from build123d import *

# Parameters (mm, degrees)
EXTRUDE_1_DEPTH     = 300
SKETCH_2_R          = 3
CUT_EXTRUDE_1_DEPTH = 4.5
SKETCH_5_R          = 1.75
CUT_EXTRUDE_2_DEPTH = 8


with BuildPart() as part:
    # 草图1 → 凸台-拉伸1 (new body)
    with BuildSketch(Plane.XY):
        Polygon((-76.761429644, 75.303838363), (-65.473589828, 75.303838363), (-65.117509736, 74.540222142), (-66.549305548, 73.537667921), (-66.549305548, 73.146885775), (-65.117509736, 72.144331554), (-65.117509736, 67.303838363), (-77.117509736, 67.303838363), (-77.117509736, 72.144331554), (-75.685713923, 73.146885775), (-75.685713923, 73.537667921), (-77.117509736, 74.540222142), align=None)
    extrude(amount=EXTRUDE_1_DEPTH)

    # 草图2 → 切除-拉伸1 (cut)
    with BuildSketch(Plane(origin=(0, 75.303838363, 0), x_dir=(1, 0, 0), z_dir=(0, 1, 0))):
        with Locations(Location((-71.117509736, -13.578086328, 0), (0, 0, 270))):
            Circle(SKETCH_2_R)
        with Locations(Location((-71.117509736, -38.578086328, 0), (0, 0, 270))):
            Circle(SKETCH_2_R)
        with Locations(Location((-71.117509736, -63.578086328, 0), (0, 0, 270))):
            Circle(SKETCH_2_R)
        with Locations(Location((-71.117509736, -88.578086328, 0), (0, 0, 270))):
            Circle(SKETCH_2_R)
        with Locations(Location((-71.117509736, -113.578086328, 0), (0, 0, 270))):
            Circle(SKETCH_2_R)
        with Locations(Location((-71.117509736, -138.578086328, 0), (0, 0, 270))):
            Circle(SKETCH_2_R)
        with Locations(Location((-71.117509736, -163.578086328, 0), (0, 0, 270))):
            Circle(SKETCH_2_R)
        with Locations(Location((-71.117509736, -188.578086328, 0), (0, 0, 270))):
            Circle(SKETCH_2_R)
        with Locations(Location((-71.117509736, -213.578086328, 0), (0, 0, 270))):
            Circle(SKETCH_2_R)
        with Locations(Location((-71.117509736, -238.578086328, 0), (0, 0, 270))):
            Circle(SKETCH_2_R)
        with Locations(Location((-71.117509736, -263.578086328, 0), (0, 0, 270))):
            Circle(SKETCH_2_R)
        with Locations(Location((-71.117509736, -288.578086328, 0), (0, 0, 270))):
            Circle(SKETCH_2_R)
    extrude(amount=-CUT_EXTRUDE_1_DEPTH, mode=Mode.SUBTRACT)

    # 草图5 → 切除-拉伸2 (cut)
    with BuildSketch(Plane(origin=(0, 75.303838363, 0), x_dir=(1, 0, 0), z_dir=(0, 1, 0))):
        with Locations(Location((-71.117509736, -13.578086328, 0), (0, 0, 270))):
            Circle(SKETCH_5_R)
        with Locations(Location((-71.117509736, -38.578086328, 0), (0, 0, 270))):
            Circle(SKETCH_5_R)
        with Locations(Location((-71.117509736, -63.578086328, 0), (0, 0, 270))):
            Circle(SKETCH_5_R)
        with Locations(Location((-71.117509736, -88.578086328, 0), (0, 0, 270))):
            Circle(SKETCH_5_R)
        with Locations(Location((-71.117509736, -113.578086328, 0), (0, 0, 270))):
            Circle(SKETCH_5_R)
        with Locations(Location((-71.117509736, -138.578086328, 0), (0, 0, 270))):
            Circle(SKETCH_5_R)
        with Locations(Location((-71.117509736, -163.578086328, 0), (0, 0, 270))):
            Circle(SKETCH_5_R)
        with Locations(Location((-71.117509736, -188.578086328, 0), (0, 0, 270))):
            Circle(SKETCH_5_R)
        with Locations(Location((-71.117509736, -213.578086328, 0), (0, 0, 270))):
            Circle(SKETCH_5_R)
        with Locations(Location((-71.117509736, -238.578086328, 0), (0, 0, 270))):
            Circle(SKETCH_5_R)
        with Locations(Location((-71.117509736, -263.578086328, 0), (0, 0, 270))):
            Circle(SKETCH_5_R)
        with Locations(Location((-71.117509736, -288.578086328, 0), (0, 0, 270))):
            Circle(SKETCH_5_R)
    extrude(amount=-CUT_EXTRUDE_2_DEPTH, mode=Mode.SUBTRACT)


solid = part.part
Here's how the part is built. I have some questions about the finished solid (model axes, mm). A direction names the side the tool comes from. Round coordinates to 2 decimals unless told otherwise and drop trailing zeros. Order: outer loops, then holes, each group sorted by start corner. A loop starts at its lowest first (then second) coordinate and runs counter-clockwise, first axis right, second up. Notation, with made-up numbers: M 35.5,89 L 43.5,89 A25 cw 43.5,112 Z; hole C 46.5,-19 d7. An arc over 180 degrees is marked long. Return JSON: item names as keys, results as strings. Group by question number.
1. If we mould it in two halves opening along X, with no side actions, what happens to faces 1 (the face through (-71, 75.304, 148)), 2 (the face through (-73, 70.804, 89))? For each: pulls with the +X half, pulls with the -X half, needs draft (parallel to the pull), parting line crosses it, or undercut.
2. If we section it at A-A on z = 99.5: List the corners of the cut face in (x, y) for me.
3. Please list where these lines run through material, in increasing order: probe 1 along X at (y, z) = (73.5, 105.5); probe 2 along X at (y, z) = (73, 38); probe 3 along Y at (x, z) = (-66.25, 93).
4. On a 3-axis mill with a long thin cutter (end or side, diameter ignored), from which of +Z, -Z, +X, -X, +Y, -Y can I reach the whole of each face in a straight line? I mean faces 3 (the face through (-70.99, 73.09, 185.58)), 4 (the face through (-71, 67.304, 148)). Say none if no direction works.
5. If we section it at B-B on y = 69: State how many separate pieces and enclosed holes the cut face has, then the cut area to 3 significant figures.
6. I'm going to push flat-ended pins straight in: pin 1 Ø5.5 at (x, z) = (-71.12, 163.58) entering from +Y; pin 2 Ø6.5 at (x, z) = (-70, 163) entering from +Y; pin 3 Ø1 at (y, z) = (74, 188.5) entering from +X. Where does each tip first touch, or does it pass through?
Reply:
{
 "1": {"face 1": "needs draft", "face 2": "undercut"},
 "2": {"outline": "M -77.12,67.3 L -65.12,67.3 L -65.12,72.14 L -66.55,73.15 L -66.55,73.54 L -65.12,74.54 L -65.47,75.3 L -76.76,75.3 L -77.12,74.54 L -75.69,73.54 L -75.69,73.15 L -77.12,72.14 Z"},
 "3": {"probe 1": "-75.69 to -66.55", "probe 2": "-75.9 to -74.06, -68.17 to -66.34", "probe 3": "67.3 to 72.94, 73.75 to 75.3"},
 "4": {"face 3": "+Y", "face 4": "+Z, -Z, +X, -X, -Y"},
 "5": {"separate pieces": "1", "enclosed holes": "12", "area": "3,480 mm^2"},
 "6": {"pin 1": "y = 70.8", "pin 2": "y = 75.3", "pin 3": "x = -65.17"}
}
